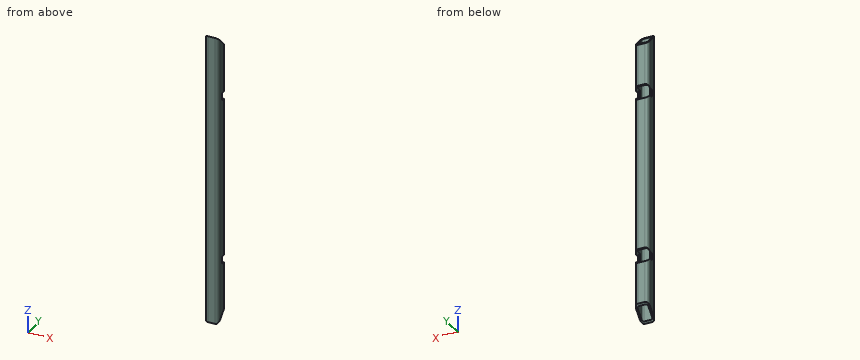
Autodesk Inventor part; units mm, degrees
ref_plane "Start plane" through (0, 0, -12.5) normal (0, 0, 1) x (1, 0, 0)
ref_plane "End plane" through (0, 0, 512.5) normal (0, 0, 1) x (1, 0, 0)
ref_plane "Work Plane4" through (0, 0, 512.5) normal (0, 0, 1) x (1, 0, 0)
ref_plane "Start plane" through (0, 0, -12.5) normal (0, 0, 1) x (1, 0, 0)
ref_plane "End plane" through (0, 0, 512.5) normal (0, 0, 1) x (1, 0, 0)
sketch "Sketch" plane through (0, 0, 0) normal (0, 0, 1) x (1, 0, 0)
  line L0 (-12.5, -6.5) -> (-12.5, 6.5)
  line L1 (-6.5, 12.5) -> (6.5, 12.5)
  line L2 (12.5, 6.5) -> (12.5, -6.5)
  line L3 (6.5, -12.5) -> (-6.5, -12.5)
  arc A0 (-12.5, -6.5) -> (-6.5, -12.5) centre (-6.5, -6.5) ccw
  arc A1 (-6.5, 12.5) -> (-12.5, 6.5) centre (-6.5, 6.5) ccw
  arc A2 (12.5, 6.5) -> (6.5, 12.5) centre (6.5, 6.5) ccw
  arc A3 (6.5, -12.5) -> (12.5, -6.5) centre (6.5, -6.5) ccw
  arc A4 (-6.5, 9.5) -> (-9.5, 6.5) centre (-6.5, 6.5) ccw
  line L4 (-6.5, 9.5) -> (6.5, 9.5)
  arc A5 (9.5, 6.5) -> (6.5, 9.5) centre (6.5, 6.5) ccw
  line L5 (9.5, 6.5) -> (9.5, -6.5)
  arc A6 (6.5, -9.5) -> (9.5, -6.5) centre (6.5, -6.5) ccw
  line L6 (6.5, -9.5) -> (-6.5, -9.5)
  arc A7 (-9.5, -6.5) -> (-6.5, -9.5) centre (-6.5, -6.5) ccw
  line L7 (-9.5, -6.5) -> (-9.5, 6.5)
  line L8 (0, 19.2397) -> (0, -19.2397) construction
  line L9 (-19.2397, 0) -> (19.2397, 0) construction
  dimension "d7" = 6
  dimension "d10" = 25
  dimension "d11" = 25
  dimension "d12" = 3
  dimension "d15" = 12.5
  dimension "d16" = 12.5
extrude "Body" add sketch "Sketch" along normal up to surface (525 mm away) from surface at -12.5
sketch "Sketch3" plane through (0, 0, 0) normal (0, 0, 1) x (1, 0, 0)
  line L0 (0, 0) -> (10, 0)
ref_plane "Work Plane3" through (0, 0, 0) normal (0, -1, 0) x (1, 0, 0)
sketch "Sketch4" plane through (0, 0, 0) normal (0, -1, 0) x (1, 0, 0)
  line L0 (-2, -12.5) -> (12, -12.5)
  line L1 (-2, 512.5) -> (12, 512.5)
  dimension "d18" = 525
ref_plane "Work Plane4" through (0, 0, 512.5) normal (0, 0, 1) x (1, 0, 0)
split "Split1" plane through (0, 0, 512.5) removes the side toward (0, 0, 1)
ref_plane "Work Plane5" through (0, -12.5, -12.5) normal (0, 0.7071, -0.7071) x (1, 0, 0)
split "Split2" plane through (0, -12.5, -12.5) removes the side toward (0, 0.7071, -0.7071)
ref_plane "Work Plane6" through (0, -12.5, 512.5) normal (0, 0.7071, 0.7071) x (1, 0, 0)
split "Split3" plane through (0, -12.5, 512.5) removes the side toward (0, 0.7071, 0.7071)
ref_plane "Work Plane7" through (0, 0, 100) normal (0, 1, 0) x (1, 0, 0)
ref_plane "Work Plane8" through (0, 800, 100) normal (0, 1, 0) x (1, 0, 0)
ref_plane "Work Plane9" through (0, 400, 100) normal (0, 1, 0) x (1, 0, 0)
sketch "Sketch5" plane through (0, 400, 100) normal (0, 1, 0) x (1, 0, 0)
  arc A0 (-12.5, -6.5) -> (-6.5, -12.5) centre (-6.5, -6.5) ccw
  line L0 (-12.5, -6.5) -> (-12.5, 6.5)
  arc A1 (-6.5, 12.5) -> (-12.5, 6.5) centre (-6.5, 6.5) ccw
  line L1 (-6.5, 12.5) -> (6.5, 12.5)
  arc A2 (12.5, 6.5) -> (6.5, 12.5) centre (6.5, 6.5) ccw
  line L2 (12.5, 6.5) -> (12.5, -6.5)
  arc A3 (6.5, -12.5) -> (12.5, -6.5) centre (6.5, -6.5) ccw
  line L3 (6.5, -12.5) -> (-6.5, -12.5)
  arc A4 (-6.5, 9.5) -> (-9.5, 6.5) centre (-6.5, 6.5) ccw
  line L4 (-6.5, 9.5) -> (6.5, 9.5)
  arc A5 (9.5, 6.5) -> (6.5, 9.5) centre (6.5, 6.5) ccw
  line L5 (9.5, 6.5) -> (9.5, -6.5)
  arc A6 (6.5, -9.5) -> (9.5, -6.5) centre (6.5, -6.5) ccw
  line L6 (6.5, -9.5) -> (-6.5, -9.5)
  arc A7 (-9.5, -6.5) -> (-6.5, -9.5) centre (-6.5, -6.5) ccw
  line L7 (-9.5, -6.5) -> (-9.5, 6.5)
extrude "Extrusion2" cut sketch "Sketch5" along normal up to surface (800 mm away) from surface at -400 contours L0 A1 L1 A2 L2 A3 L3 A0 | L4 A5 L5 A6 L6 A7 L7 A4
ref_plane "Work Plane10" through (0, 800, 400) normal (0, -1, 0) x (-1, 0, 0)
ref_plane "Work Plane11" through (0, 0, 400) normal (0, -1, 0) x (-1, 0, 0)
ref_plane "Work Plane12" through (0, 400, 400) normal (0, -1, 0) x (-1, 0, 0)
sketch "Sketch6" plane through (0, 400, 400) normal (0, -1, 0) x (-1, 0, 0)
  arc A0 (-12.5, -6.5) -> (-6.5, -12.5) centre (-6.5, -6.5) ccw
  line L0 (-12.5, -6.5) -> (-12.5, 6.5)
  arc A1 (-6.5, 12.5) -> (-12.5, 6.5) centre (-6.5, 6.5) ccw
  line L1 (-6.5, 12.5) -> (6.5, 12.5)
  arc A2 (12.5, 6.5) -> (6.5, 12.5) centre (6.5, 6.5) ccw
  line L2 (12.5, 6.5) -> (12.5, -6.5)
  arc A3 (6.5, -12.5) -> (12.5, -6.5) centre (6.5, -6.5) ccw
  line L3 (6.5, -12.5) -> (-6.5, -12.5)
  arc A4 (-6.5, 9.5) -> (-9.5, 6.5) centre (-6.5, 6.5) ccw
  line L4 (-6.5, 9.5) -> (6.5, 9.5)
  arc A5 (9.5, 6.5) -> (6.5, 9.5) centre (6.5, 6.5) ccw
  line L5 (9.5, 6.5) -> (9.5, -6.5)
  arc A6 (6.5, -9.5) -> (9.5, -6.5) centre (6.5, -6.5) ccw
  line L6 (6.5, -9.5) -> (-6.5, -9.5)
  arc A7 (-9.5, -6.5) -> (-6.5, -9.5) centre (-6.5, -6.5) ccw
  line L7 (-9.5, -6.5) -> (-9.5, 6.5)
extrude "Extrusion3" cut sketch "Sketch6" along normal up to surface (800 mm away) from surface at -400 contours L0 A1 L1 A2 L2 A3 L3 A0 | L4 A5 L5 A6 L6 A7 L7 A4
equation "\"d7\" = G_IR"
equation "\"d10\" = G_H"
equation "\"d11\" = G_W"
equation "\"d12\" = G_T"
equation "\"d15\" = 0.5 * d10"
equation "\"d16\" = 0.5 * d11"
equation "\"d3\" = G_L"
equation "\"G_W\" = 25"
equation "\"G_H\" = 25"
equation "\"G_T\" = 3"
equation "\"G_IR\" = 6"
equation "\"G_L\" = d18"
equation "\"G_OFFSET_START\" = 12.5"
equation "\"G_OFFSET_END\" = 12.5"
equation "\"d13\" = -G_OFFSET_START"
equation "\"d14\" = G_OFFSET_END + B_L"
properties part number "AS 1163 - C350L0 25x25x3.0 SHS - 525" material "Steel, Mild"
Work out the finished part from the listing and answer in its coordinate system (mm). Coordinates: 2 decimals unless noted, no trailing zeros. Write each loop counter-clockwise with the first axis right and the second up, starting at its lowest first coordinate (ties: lowest second). Pieces come first, ordered by that corner, then holes. Notation, with made-up numbers: M 84.25,-4 L 131.25,-4 A20 cw 131.25,13 Z; hole C -23,-33.5 d11. An arc over 180 degrees is marked long. Use one line per item in the form item = value. Start each with the question number.
1. The part is cut by section B-B (z = 100). Give the vertices of the cut face in (x, y), plus the area to 3 significant figures.
2. Each of these flat-tipped pins is pushed along its axis until it touches: P1, Ø0.9, axis at x = -3, y = 11, coming from the -Z side; P2, Ø1.5, axis at x = 1, y = 11.5, coming from the +Z side; P3, Ø4, axis at x = 9, z = 285.5, coming from the -Y side. Where does it stop, or does it pass through?
3. The part is cut by section A-A (z = 280). Give the vertices of the cut face in (x, y).
4. Straight lines are drawn through the part: probe 1 along X at (y, z) = (-4, 348.5); probe 2 along Y at (x, z) = (7, 193.5); probe 3 along Z at (x, y) = (9.75, 3). For each, find the intervals that lie inside material, in ascending order. Write a range as from..to.
Evaluation:
q1.outline = M -12.5,-6.5 A6 ccw -6.5,-12.5 L 6.5,-12.5 A6 ccw 12.5,-6.5 L 12.5,0 L 9.5,0 L 9.5,-6.5 A3 cw 6.5,-9.5 L -6.5,-9.5 A3 cw -9.5,-6.5 L -9.5,0 L -12.5,0 Z
q1.area = 120 mm^2
q2.P1 = 10.55
q2.P2 = 489.25
q2.P3 = -12.48
q3.outline = M -12.5,-6.5 A6 ccw -6.5,-12.5 L 6.5,-12.5 A6 ccw 12.5,-6.5 L 12.5,6.5 A6 ccw 6.5,12.5 L -6.5,12.5 A6 ccw -12.5,6.5 Z; hole M -9.5,-6.5 A3 ccw -6.5,-9.5 L 6.5,-9.5 A3 ccw 9.5,-6.5 L 9.5,6.5 A3 ccw 6.5,9.5 L -6.5,9.5 A3 ccw -9.5,6.5 Z
q4.probe_1 = -12.5..-9.5, 9.5..12.5
q4.probe_2 = -12.48..-9.46, 9.46..12.48
q4.probe_3 = 3..88.46, 111.54..388.46, 411.54..497
